The model under review builds one solid part; all positions refer to its coordinate system, in mm. Face numbers are marked on the shaded views. Round coordinates to 2 decimals unless told otherwise and drop trailing zeros. Loops run counter-clockwise (first coordinate to the right, second up) from the corner with the lowest first, then second, coordinate; pieces in that order, holes last. Notation, with made-up numbers: M 44,29.5 L 50,29.5 A21 cw 50,42.5 Z; hole C 53,17.5 d11. An arc over 180 degrees is marked long. Answer as a JSON object with one key per item and string values. Group by question number.
Item 1: Consider section B-B (z = 0.7). Give the boundary of the cut face in (x, y).
Item 2: To check wall thickness, follow line 1 (Y direction, x = 0, z = 1); line 2 (X direction, y = 38, z = 4.3); line 3 (Y direction, x = -2.25, z = 4.5). State the ranges of each line that lie inside material, in increasing order.
Item 3: The part is to be moulded in two halves that separate along X. For the marked faces 1, 2, 3 and 4, say which applies: +X half, -X half, draft (parallel to the pull), parting line (faces both ways), or undercut.
Item 4: Consider section C-C (y = 61). Give the boundary of the cut face in (x, z), and give its area (3 significant figures).
Item 5: Consider section D-D (y = 12.7). Give the boundary of the cut face in (x, z), and give its area (3 significant figures).
Item 6: Consider section A-A (x = 0). Give the boundary of the cut face in (y, z), and give its area (3 significant figures).
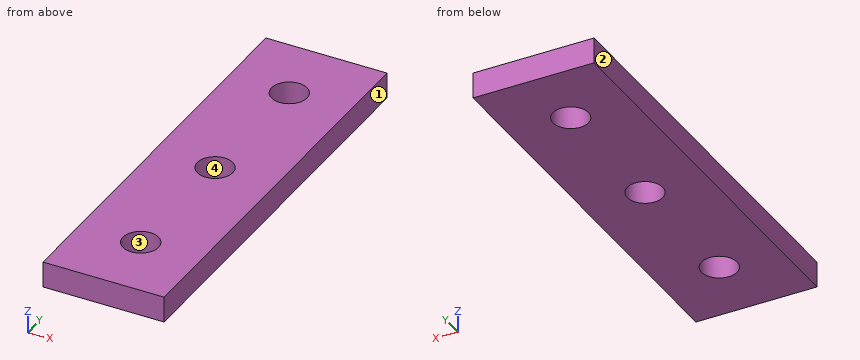
Autodesk Inventor part; units mm, degrees
ref_plane "YZ Plane" through (0, 0, 0) normal (1, 0, 0) x (0, 1, 0)
ref_plane "XZ Plane" through (0, 0, 0) normal (0, 1, 0) x (-1, 0, 0)
ref_plane "XY Plane" through (0, 0, 0) normal (0, 0, 1) x (1, 0, 0)
sketch "Sketch_1" plane through (0, 0, 0) normal (0, 0, 1) x (1, 0, 0)
  line L0 (-11.1125, 76.2) -> (-11.1125, 0)
  line L1 (-11.1125, 0) -> (11.1125, 0)
  line L2 (11.1125, 0) -> (11.1125, 76.2)
  line L3 (11.1125, 76.2) -> (-11.1125, 76.2)
  circle A0 centre (0, 12.7) radius 3.2639
  circle A1 centre (0, 38.1) radius 3.2639
  circle A2 centre (0, 63.5) radius 3.2639
extrude "Extrusion1" add sketch "Sketch_1" along normal blind 4.7752
properties part number "4118"
Geometry results:
{
 "1": {"outline": "M -11.11,0 L 11.11,0 L 11.11,76.2 L -11.11,76.2 Z; hole C 0,12.7 d6.53; hole C 0,38.1 d6.53; hole C 0,63.5 d6.53"},
 "2": {"line 1": "y = 0 to 9.44, 15.96 to 34.84, 41.36 to 60.24, 66.76 to 76.2", "line 2": "x = -11.11 to -3.26, 3.26 to 11.11", "line 3": "y = 0 to 10.34, 15.06 to 35.74, 40.46 to 61.14, 65.86 to 76.2"},
 "3": {"face 1": "+X half", "face 2": "-X half", "face 3": "undercut", "face 4": "undercut"},
 "4": {"outline": "M -11.11,0 L -2.1,0 L -2.1,4.78 L -11.11,4.78 Z; M 2.1,0 L 11.11,0 L 11.11,4.78 L 2.1,4.78 Z", "area": "86.1 mm^2"},
 "5": {"outline": "M -11.11,0 L -3.26,0 L -3.26,4.78 L -11.11,4.78 Z; M 3.26,0 L 11.11,0 L 11.11,4.78 L 3.26,4.78 Z", "area": "75.0 mm^2"},
 "6": {"outline": "M 0,0 L 9.44,0 L 9.44,4.78 L 0,4.78 Z; M 15.96,0 L 34.84,0 L 34.84,4.78 L 15.96,4.78 Z; M 41.36,0 L 60.24,0 L 60.24,4.78 L 41.36,4.78 Z; M 66.76,0 L 76.2,0 L 76.2,4.78 L 66.76,4.78 Z", "area": "270 mm^2"}
}
